Answer from the drawing. Dimensions are ordinates in mm from the lowest x, y and z of the part. A direction names the side the tool comes from. Round coordinates to 2 decimals unless told otherwise and drop trailing zeros.
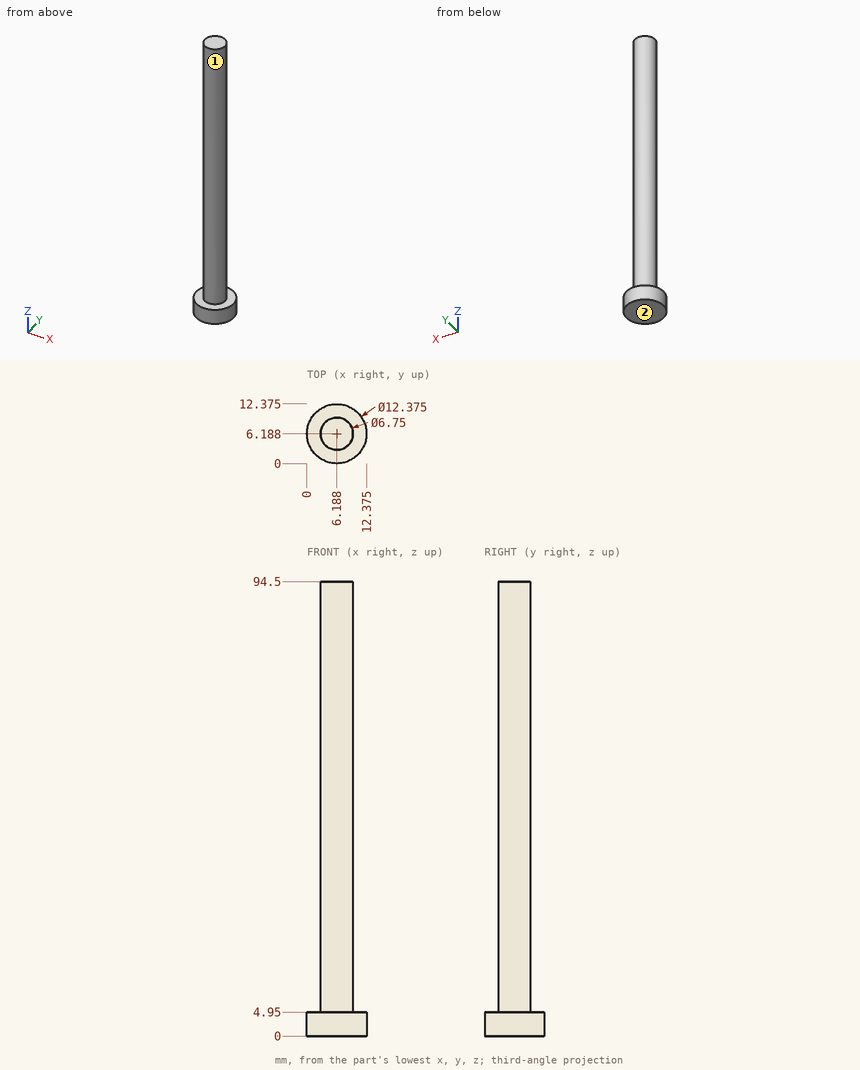
Item 1: For the marked faces 1 and 2, determine the directions among +Z, -Z, +X, -X, +Y, -Y from which every point of the face is accessible in a straight line to the end or side of a thin tool.
Item 2: Straight lines are drawn through the part: line 1 (Z direction, x = 2.5, y = 4); line 2 (X direction, y = 6.5, z = 12.5); line 3 (Y direction, x = 6.25, z = 74). For each, find the intervals that lie inside material, in ascending order.
Item 3: Each of these flat-tipped pins is pushed along its axis until it touches: P1, Ø2, axis at x = 8, z = 14, coming from the +Y side; P2, Ø1, axis at x = 4, z = 73, coming from the -Y side (1 decimal); P3, Ø1.5, axis at x = 9, z = 61.5, coming from the -Y side (1 decimal). Where does it stop, or does it pass through?
Answer below:
1. face 1: +Z
1. face 2: -Z, +X, -X, +Y, -Y
2. line 1: z = 0 to 4.95
2. line 2: x = 2.83 to 9.55
2. line 3: y = 2.81 to 9.56
3. P1: stops at y = 9.46
3. P2: stops at y = 3.3
3. P3: stops at y = 3.5
